Geometry check sheet. Reference: the model listing, model coordinates, mm. Face numbers are marked on the shaded views. A direction names the side the tool comes from. Give positions to 0.01 mm unless a question says otherwise; leave off trailing zeros. Order: outer loops, then holes, each group sorted by start corner. A loop starts at its lowest first (then second) coordinate and runs counter-clockwise, first axis right, second up. Notation, with made-up numbers: M 11.5,23.5 L 22.5,23.5 A24 ccw 22.5,62.5 Z; hole C -17.75,14 d1. An arc over 180 degrees is marked long. Use CSV: the item, a comma, the result in double quotes. Start each with the question number.
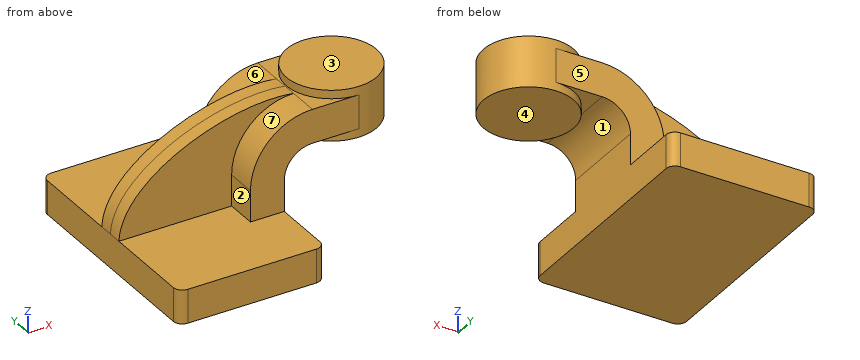
from build123d import *

# Parameters (mm, degrees)
F1_DEPTH = 63.5
F2_DEPTH = 25.4
F3_DEPTH = 7.9375
F5_R     = 5.08


# Not quite as in the source:
# - ends of sketch curves that miss each other by under 0.0002 mm in the source are joined


with BuildPart() as f1:
    # F0 (on Front) → F1 (new body, symmetric)
    with BuildSketch(Plane.XZ):
        Polygon((41.275, -9.525), (41.275, 9.525), (22.225, 9.525), (-41.275, 9.525), (-41.275, -9.525), align=None)
    extrude(amount=F1_DEPTH, both=True)

    # F0 (on Front) → F2 (join, symmetric)
    with BuildSketch(Plane.XZ):
        with BuildLine():
            Line((22.225, 9.525), (41.275, 9.525))
            Line((41.275, 9.525), (41.275, 27.0002))
            ThreePointArc((41.275, 27.0002), (45.9246798487, 38.2255201513), (57.15, 42.8752))
            Line((57.15, 42.8752), (57.8334331512, 42.8752))
            Line((57.8334331512, 42.8752), (57.8334331512, 61.9252))
            Line((57.8334331512, 61.9252), (57.15, 61.9252))
            ThreePointArc((57.15, 61.9252), (32.4542956671, 51.6959043329), (22.225, 27.0002))
            Line((22.225, 27.0002), (22.225, 9.525))
        make_face()
        Polygon((57.8334331512, 61.9252), (57.8334331512, 42.8752), (83.2334309816, 42.8752), (83.2334331512, 61.9252), align=None)
    extrude(amount=F2_DEPTH, both=True)

    # F0 (on Front) → F3 (join, symmetric)
    with BuildSketch(Plane.XZ):
        with BuildLine():
            Line((-41.275, 9.525), (22.225, 9.525))
            Line((22.225, 9.525), (22.225, 27.0002))
            ThreePointArc((22.225, 27.0002), (32.4542956671, 51.6959043329), (57.15, 61.9252))
            add(Edge.make_bspline(
                [(-41.275, 9.525), (-39.7025756538, 42.9233573377), (20.2414225787, 67.5613582134), (57.15, 61.9252)],
                knots=[0, 0, 0, 0, 111.5045361635, 111.5045361635, 111.5045361635, 111.5045361635], degree=3))
        make_face()
    extrude(amount=F3_DEPTH, both=True)

    # F0 (on Front) → F4 (revolve)
    with BuildSketch(Plane.XZ):
        Polygon((83.2334331512, 61.9252), (83.2334331512, 42.8752), (83.2334331512, 38.1), (108.6334331512, 38.1), (108.6334331512, 66.675), (83.2334331512, 66.675), align=None)
    revolve(axis=Axis((83.2334331512, 0, 52.3875), (0, 0, 1)))

    # F5
    f5_edges = [f1.edges().sort_by_distance(p)[0] for p in [
        (-41.275, -63.5, 0),
        (41.275, -63.5, 0),
        (-41.275, 63.5, 0),
        (41.275, 63.5, 0),
    ]]
    fillet(f5_edges, radius=F5_R)


solid = f1.part
(1) Sectioned sample at A-A on z = -1. Record the cut outline in (x, y) (3 decimals).
(2) Sectioned sample at D-D on x = 86. Record the cut outline in (y, z) (3 decimals), then the cut area to 3 significant figures.
(3) Go/stop test with flat-tipped pins: P1, Ø21, axis at x = 73, y = -10.5, coming from the -Z side; P2, Ø11, axis at y = -7.5, z = 1.5, coming from the +X side (3 decimals); P3, Ø4, axis at x = 25, z = 43.5, coming from the -Y side; P4, Ø2, axis at y = -32.5, z = 12, coming from the -X side. Record where each tip stops, or that it passes through.
(4) Sectioned sample at B-B on y = -17. Record the cut outline in (x, z) (3 decimals), then the cut area to 3 significant figures.
(5) Access from +Z, -Z, +X, -X, +Y, -Y to the whole of each face (thin tool, end or side, straight path). Record for the marked faces 4, 5, 6 and 7.
(6) Sectioned sample at C-C on x = 67. Record the cut outline in (y, z) (1 decimal).
(7) Thickness scan on line 1 (Z direction, x = -17.5, y = 57) (3 decimals); line 2 (X direction, y = 17.5, z = 13.5) (3 decimals); line 3 (Y direction, x = 38.5, z = 60). Record the ranges inside material, lowest first.
(8) Draft check along X on the marked faces 1, 2 and 3. Enter one of: +X half, -X half, draft (parallel to the pull), parting line (faces both ways), or undercut.
Responses:
1,outline,"M -41.275,-58.42 A5.08 ccw -36.195,-63.5 L 36.195,-63.5 A5.08 ccw 41.275,-58.42 L 41.275,58.42 A5.08 ccw 36.195,63.5 L -36.195,63.5 A5.08 ccw -41.275,58.42 Z"
2,outline,"M -25.249,38.1 L 25.249,38.1 L 25.249,66.675 L -25.249,66.675 Z"
2,area,"1,440 mm2"
3,P1,"z = 38.1"
3,P2,"x = 41.275"
3,P3,"y = -25.4"
3,P4,"through"
4,outline,"M -41.275,-9.525 L 41.275,-9.525 L 41.275,27 A15.875 cw 57.15,42.875 L 64.361,42.875 L 64.361,38.1 L 102.106,38.1 L 102.106,66.675 L 64.361,66.675 L 64.361,61.925 L 57.15,61.925 A34.925 ccw 22.225,27 L 22.225,9.525 L -41.275,9.525 Z"
4,area,"3,880 mm2"
5,face 4,"-Z, +X, +Y, -Y"
5,face 5,"+Z, +X, -X, +Y"
5,face 6,"+Z, -X, +Y"
5,face 7,"+Z, -X, -Y"
6,outline,"M -25.4,42.9 L -19.5,42.9 L -19.5,38.1 L 19.5,38.1 L 19.5,42.9 L 25.4,42.9 L 25.4,61.9 L 19.5,61.9 L 19.5,66.7 L -19.5,66.7 L -19.5,61.9 L -25.4,61.9 Z"
7,line 1,"-9.525 to 9.525"
7,line 2,"22.225 to 41.275"
7,line 3,"-7.94 to 7.94"
8,face 1,"undercut"
8,face 2,"-X half"
8,face 3,"draft"
